Read the model definition and answer for the solid it produces. Units are mm, in the model's axes. A direction names the side the tool comes from. Give positions to 0.01 mm unless a question says otherwise; leave off trailing zeros. Order: outer loops, then holes, each group sorted by start corner. A loop starts at its lowest first (then second) coordinate and runs counter-clockwise, first axis right, second up.
Item 1: A cutting plane is placed at D-D (y = -14.5). Write down the section's boundary in (x, z), plus the area to 3 significant figures.
Item 2: A cutting plane is placed at C-C (z = 19). Write down the section's boundary in (x, y) (3 decimals), plus the area to 3 significant figures.
Item 3: A cutting plane is placed at B-B (x = 0). Write down the section's boundary in (y, z).
Item 4: Given pin 1 Ø0.8 at (x, y) = (7, -23) entering from +Z; pin 2 Ø0.5 at (x, z) = (6.5, 4.5) entering from -Y; pin 3 Ø12 at (y, z) = (11, 9) entering from -X; pin 4 Ø20.5 at (x, y) = (0, 0) entering from +Z, each flat-ended and moving along its own axis, determine where each tip first touches the part or whether it passes through.
Item 5: A cutting plane is placed at A-A (y = 0). Write down the section's boundary in (x, z), plus the area to 3 significant figures.
Item 6: Which of the six approach directions +Z, -Z, +X, -X, +Y, -Y give full straight-line access (tool end or side, diameter ignored) to faces 4 (the face through (11.842, -23, 19)), 5 (the face through (0.93, 23.73, 18.78)), 6 (the face through (-1, -22.363, 25)), 7 (the face through (0.4, -20.6, 1.1))?
Item 7: The mould has two halves that part along X. Classify faces 1 (the face through (-7, -23, 3.1)), 2 (the face through (-11, -9, 38.1)), 3 (the face through (-11.949, -23, 19)): +X half, -X half, draft (parallel to the pull), parting line (faces both ways), or undercut.
Item 8: Find the intervals of material crossed by line 1 along Y through (x, z) = (0, 27); line 2 along Y through (x, z) = (7.5, 35); line 3 along Z through (x, y) = (0, -16), in increasing order.
from build123d import *

# Parameters (mm, degrees)
SKETCH1_R               = 12.824135806
BOSS_EXTRUDE2_DEPTH     = 38.1
CUT_EXTRUDE1_DEPTH      = 35
CUT_EXTRUDE2_DEPTH      = 23.57
CUT_EXTRUDE2_DEPTH_BACK = 23.57
SKETCH6_R               = 8


with BuildPart() as part:
    # Sketch1 → Boss-Extrude2 (new body)
    with BuildSketch(Plane.XY):
        with BuildLine():
            Line((11.842048876, -25.66709252), (11.842048876, -20.58709252))
            ThreePointArc((11.842048876, -20.58709252), (0.061981133, 23.749919123), (-11.94934079, -20.525003159))
            Line((-11.94934079, -20.525003159), (-11.94934079, -25.605003159))
            ThreePointArc((-11.94934079, -25.605003159), (-0.067090695, -30.787800341), (11.842048876, -25.66709252))
        make_face()
        with Locations(Location((0, 0, 0), (0, 0, 180))):
            Circle(SKETCH1_R, mode=Mode.SUBTRACT)
    extrude(amount=BOSS_EXTRUDE2_DEPTH)

    # Sketch3 → Cut-Extrude1 (cut)
    with BuildSketch(Plane.XY.offset(38.1)):
        with BuildLine():
            Line((-8.95388159, -22.363138181), (7.04611841, -22.363138181))
            ThreePointArc((7.04611841, -22.363138181), (7.80811841, -23.125138181), (7.04611841, -23.887138181))
            Line((7.04611841, -23.887138181), (-8.95388159, -23.887138181))
            ThreePointArc((-8.95388159, -23.887138181), (-9.71588159, -23.125138181), (-8.95388159, -22.363138181))
        make_face()
    extrude(amount=-CUT_EXTRUDE1_DEPTH, mode=Mode.SUBTRACT)

    # Sketch6 → Cut-Extrude2 (cut, two sides: drawn at the far end of the back side and taken through both)
    with BuildSketch(Plane(origin=(0, -23.887138181, 0), x_dir=(1, 0, 0), z_dir=(0, 1, 0)).offset(-CUT_EXTRUDE2_DEPTH_BACK)):
        with Locations(Location((0, -9.09196145, 0), (0, 0, 270))):
            Circle(SKETCH6_R)
    extrude(amount=CUT_EXTRUDE2_DEPTH + CUT_EXTRUDE2_DEPTH_BACK, mode=Mode.SUBTRACT)


solid = part.part
Response values:
1. outline: (-18.81, 0) - (18.81, 0) - (18.81, 38.1) - (-18.81, 38.1) - close; hole circle Ø16 at (0, 9.09)
1. area: 1,230 mm2
2. outline: (-11.949, -25.605) arc R16.31 ccw to (11.842, -25.667) - (11.842, -20.587) arc R23.75 ccw (long way) to (-11.949, -20.525) - close; hole circle Ø25.648 at (0, 0); hole (-8.954, -23.887) - (7.046, -23.887) arc R0.762 ccw to (7.046, -22.363) - (-8.954, -22.363) arc R0.762 ccw to start
2. area: 1,380 mm2
3. outline: (-30.79, 0) - (-12.82, 0) - (-12.82, 1.09) - (-30.79, 1.09) - close; (-30.79, 17.09) - (-23.89, 17.09) - (-23.89, 38.1) - (-30.79, 38.1) - close; (-22.36, 17.09) - (-12.82, 17.09) - (-12.82, 38.1) - (-22.36, 38.1) - close; (12.82, 0) - (23.75, 0) - (23.75, 38.1) - (12.82, 38.1) - close
4. pin 1: stops at z = 3.1
4. pin 2: stops at y = -29.47
4. pin 3: stops at x = -23.22
4. pin 4: passes through
5. outline: (-23.75, 0) - (-12.82, 0) - (-12.82, 38.1) - (-23.75, 38.1) - close; (12.82, 0) - (23.75, 0) - (23.75, 38.1) - (12.82, 38.1) - close
5. area: 833 mm2
6. face 4: +Z, -Z, +X, -Y
6. face 5: +Z, -Z
6. face 6: +Z
6. face 7: -Y
7. face 1: undercut
7. face 2: draft
7. face 3: -X half
8. line 1: y = -30.79 to -23.89, -22.36 to -12.82, 12.82 to 23.75
8. line 2: y = -28.95 to -23.74, -22.51 to -10.4, 10.4 to 22.53
8. line 3: z = 0 to 1.09, 17.09 to 38.1
